Input: part model. Units: mm. Frame: model coordinates. Round coordinates to 2 decimals unless told otherwise and drop trailing zeros. Loops run counter-clockwise (first coordinate to the right, second up) from the corner with the lowest first, then second, coordinate; pieces in that order, holes last. Notation, with made-up numbers: M 1.25,19.25 L 28.25,19.25 A12 ccw 28.25,29.25 Z; hole C -12.75,15.5 d5. An arc over 180 degrees is marked long. Put each result on its own line as item: value. Start each with the question number.
1) Line query: probe 1 along Y at (x, z) = (0, 0.7); probe 2 along Z at (x, y) = (7.25, 1); probe 3 along Y at (x, z) = (6, 1.7). Output: solid intervals per line, ascending.
2) Section C-C on z = 112. Output: boundary loops of the cut face in (x, y), plus the area to 3 significant figures.
3) Section A-A on y = 0. Output: boundary loops of the cut face in (x, z).
4) Pin query (flat end, axial travel): pin 1 (1.9 mm diameter, centred on x = 0, y = 6, fed in from +Z); pin 2 (5 mm diameter, centred on y = 3, z = 103, fed in from +X); pin 3 (2 mm diameter, centred on x = -1.5, z = 168, fed in from -Y); pin 4 (6 mm diameter, centred on y = -5.5, z = 84.5, fed in from +X). Return the tip coordinate at first contact, or that it passes through.
from build123d import *

# Parameters (mm, degrees)
SKETCH1_R           = 9
SKETCH1_R_2         = 1.55
BOSS_EXTRUDE1_DEPTH = 3
SKETCH2_R           = 3
BOSS_EXTRUDE2_DEPTH = 185


with BuildPart() as part:
    # Sketch1 → Boss-Extrude1 (new body)
    with BuildSketch(Plane.XY):
        Circle(SKETCH1_R)
        with Locations((-6, 0)):
            Circle(SKETCH1_R_2, mode=Mode.SUBTRACT)
        with Locations((0, 6)):
            Circle(SKETCH1_R_2, mode=Mode.SUBTRACT)
        with Locations((6, 0)):
            Circle(SKETCH1_R_2, mode=Mode.SUBTRACT)
        with Locations((0, -6)):
            Circle(SKETCH1_R_2, mode=Mode.SUBTRACT)
    extrude(amount=BOSS_EXTRUDE1_DEPTH)

    # Sketch2 → Boss-Extrude2 (add)
    with BuildSketch(Plane.XY.offset(3)):
        Circle(SKETCH2_R)
    extrude(amount=BOSS_EXTRUDE2_DEPTH)


solid = part.part
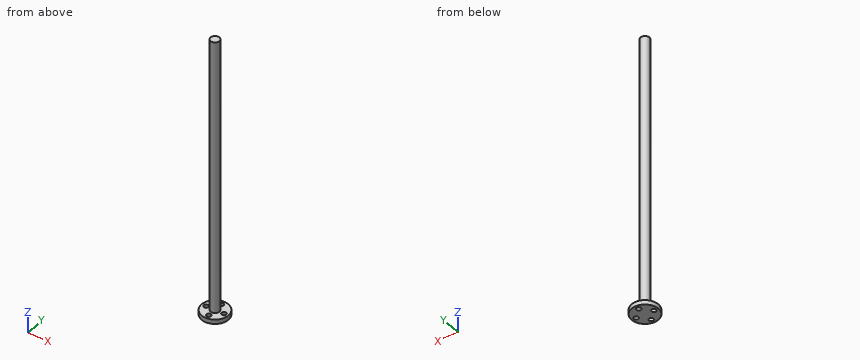
Geometry results:
1. probe 1: y = -9 to -7.55, -4.45 to 4.45, 7.55 to 9
1. probe 2: z = 0 to 3
1. probe 3: y = -6.71 to -1.55, 1.55 to 6.71
2. outline: C 0,0 d6
2. area: 28.3 mm²
3. outline: M -9,0 L -7.55,0 L -7.55,3 L -9,3 Z; M -4.45,0 L 4.45,0 L 4.45,3 L 3,3 L 3,188 L -3,188 L -3,3 L -4.45,3 Z; M 7.55,0 L 9,0 L 9,3 L 7.55,3 Z
4. pin 1: passes through
4. pin 2: stops at x = 2.96
4. pin 3: stops at y = -2.96
4. pin 4: stops at x = 1.66
